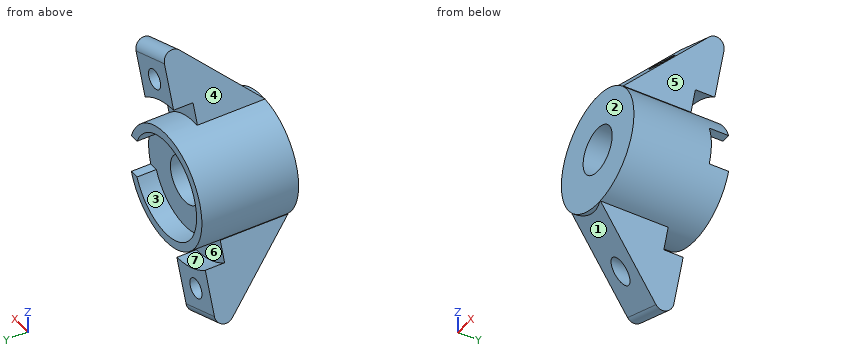
```python
from build123d import *

# Parameters (mm, degrees)
SKETCH1_R            = 12
SKETCH1_R_2          = 4.8
BOSS_EXTRUDE2_DEPTH  = 20
SKETCH1_3_R          = 4.8
CUT_EXTRUDE2_DEPTH   = 27.229754097
SKETCH3_R            = 10.25
CUT_EXTRUDE3_DEPTH   = 4
SKETCH5_W            = 11.035067707
SKETCH5_H            = 8
CUT_EXTRUDE5_DEPTH   = 4
BOSS_EXTRUDE3_DEPTH  = 5
SKETCH7_R            = 16.1
SKETCH7_R_2          = 12
CUT_EXTRUDE6_DEPTH   = 6
CUT_EXTRUDE7_REACH   = 39.1
SKETCH9_R            = 2
FILLET1_R            = 2
FILLET1_OF_MIRROR1_R = 2


with BuildPart() as part:
    # Sketch1 → Boss-Extrude2 (new body)
    # profile 1 of 2: a face of its own
    with BuildSketch(Plane(origin=(0, 0, 0), x_dir=(1, 0, 0), z_dir=(0, 1, 0))):
        with Locations(Location((0, 0, 0), (0, 0, 270))):
            Circle(SKETCH1_R)
        Circle(SKETCH1_R_2, mode=Mode.SUBTRACT)
    # profile 2 of 2: a face of its own
    with BuildSketch(Plane(origin=(0, 0, 0), x_dir=(1, 0, 0), z_dir=(0, 1, 0))):
        Circle(SKETCH1_R_2)
    extrude(amount=-BOSS_EXTRUDE2_DEPTH)

    # Sketch1<3> → Cut-Extrude2 (cut, through all)
    with BuildSketch(Plane(origin=(0, 0, 0), x_dir=(1, 0, 0), z_dir=(0, 1, 0))):
        with Locations(Location((0, 0, 0), (0, 0, 270))):
            Circle(SKETCH1_3_R)
    extrude(amount=-CUT_EXTRUDE2_DEPTH, mode=Mode.SUBTRACT)

    # Sketch3 → Cut-Extrude3 (cut)
    with BuildSketch(Plane(origin=(0, 0, 0), x_dir=(1, 0, 0), z_dir=(0, 1, 0))):
        with Locations(Location((0, 0, 0), (0, 0, 270))):
            Circle(SKETCH3_R)
    extrude(amount=-CUT_EXTRUDE3_DEPTH, mode=Mode.SUBTRACT)

    # Sketch5 → Cut-Extrude5 (cut)
    with BuildSketch(Plane(origin=(0, 0, 0), x_dir=(1, 0, 0), z_dir=(0, 1, 0))):
        with Locations((10.966087066, 0)):
            Rectangle(SKETCH5_W, SKETCH5_H)
    extrude(amount=-CUT_EXTRUDE5_DEPTH, mode=Mode.SUBTRACT)

    # Sketch6 → Boss-Extrude3 (add, symmetric)
    with BuildSketch(Plane(origin=(0, 0, 0), x_dir=(0, -1, 0), z_dir=(-0.9396926207859094, 0, 0.34202014332566616))):
        Polygon((2, -11), (20, -11), (2, -29), align=None)
    boss_extrude3 = extrude(amount=BOSS_EXTRUDE3_DEPTH, both=True)

    # Sketch7 → Cut-Extrude6 (cut)
    with BuildSketch(Plane(origin=(0, 0, 0), x_dir=(1, 0, 0), z_dir=(0, 1, 0))):
        Circle(SKETCH7_R)
        with Locations(Location((0, 0, 0), (0, 0, 340.528779366))):
            Circle(SKETCH7_R_2, mode=Mode.SUBTRACT)
    cut_extrude6 = extrude(amount=-CUT_EXTRUDE6_DEPTH, mode=Mode.SUBTRACT)

    # Cut-Extrude7: up to this plane
    cut_extrude7_end = Plane(origin=(0.936241527, -20, -12.046719545), z_dir=(-0.2418447626479747, -0.7071067811865439, -0.664463024388679))
    # Sketch9 → Cut-Extrude7 (cut, up to the surface)
    with BuildSketch(Plane(origin=(0, -2, 0), x_dir=(1, 0, 0), z_dir=(0, 1, 0)), mode=Mode.PRIVATE) as cut_extrude7_sk1:
        with Locations(Location((-6.840402867, 18.793852416, 0), (0, 0, 270))):
            Circle(SKETCH9_R)
    cut_extrude7_tool1 = split(extrude(cut_extrude7_sk1.sketch, amount=-CUT_EXTRUDE7_REACH, mode=Mode.PRIVATE), bisect_by=cut_extrude7_end, keep=Keep.BOTH, mode=Mode.PRIVATE)
    cut_extrude7 = cut_extrude7_tool1.solids().sort_by_distance((-6.840403, -2, -18.793852))[0]
    add(cut_extrude7, mode=Mode.SUBTRACT)

    # Fillet1
    fillet1_edges = [part.edges().sort_by_distance(p)[0] for p in [
        (-9.918584156, -2, -27.251086003),
    ]]
    fillet(fillet1_edges, radius=FILLET1_R)

    # Mirror1: Boss-Extrude3, Cut-Extrude6, Cut-Extrude7 across plane
    add(boss_extrude3.mirror(Plane(origin=(0, 0, 0), x_dir=(0.9396926207859094, 0, -0.3420201433256661), z_dir=(-0.3420201433256661, 0, -0.9396926207859093))))
    add(cut_extrude6.mirror(Plane(origin=(0, 0, 0), x_dir=(0.9396926207859094, 0, -0.3420201433256661), z_dir=(-0.3420201433256661, 0, -0.9396926207859093))), mode=Mode.SUBTRACT)
    add(cut_extrude7.mirror(Plane(origin=(0, 0, 0), x_dir=(0.9396926207859094, 0, -0.3420201433256661), z_dir=(-0.3420201433256661, 0, -0.9396926207859093))), mode=Mode.SUBTRACT)

    # Fillet1 of Mirror1
    fillet1_of_mirror1_edges = [part.edges().sort_by_distance(p)[0] for p in [
        (9.918584156, -2, 27.251086003),
    ]]
    fillet(fillet1_of_mirror1_edges, radius=FILLET1_OF_MIRROR1_R)


solid = part.part
```
The listing builds one solid part. Answer for the finished solid, in the listing's coordinates (mm). Face numbers are marked on the shaded views. A direction names the side the tool comes from. Coordinates: 2 decimals unless noted, no trailing zeros. Order: outer loops, then holes, each group sorted by start corner. A loop starts at its lowest first (then second) coordinate and runs counter-clockwise, first axis right, second up. Notation, with made-up numbers: M 72.25,-27.75 L 92.25,-27.75 A20 ccw 92.25,-6.75 Z; hole C -2,80 d2. An arc over 180 degrees is marked long. Answer as a JSON object with one key per item and string values. Group by question number.
1. Section D-D on z = -18 is taken. Write down the section's boundary in (x, y), then the cut area to 3 significant figures.
2. Determine the mould class of the marked faces 1, 2, 3 and 4 for opening direction Z: released by +Z, released by -Z, zero draft, split by the parting line, or undercut.
3. Straight lines are drawn through the part: line 1 (X direction, y = -13.75, z = 0); line 2 (Z direction, x = 4.5, y = -2.75); line 3 (Y direction, x = 5.75, z = -7.5). For each, find the intervals that lie inside material, in ascending order.
4. Flat-ended cylindrical pins translate along their axes: P1, Ø6.5, axis at x = 6.84, z = 18.79, coming from the -Y side; P2, Ø5, axis at y = -16, z = -17, coming from the +X side; P3, Ø1, axis at y = -12, z = 0, coming from the -X side; P4, Ø3.5, axis at x = -6.84, z = -18.79, coming from the +Y side. Find the tip coordinate at first contact, or state that the pin passes through.
5. Section B-B on x = 0 is taken. Write down the section's boundary in (y, z), then the cut area to 3 significant figures.
6. Section A-A on z = 0 is taken. Write down the section's boundary in (x, y), then the cut area to 3 significant figures.
7. A tool of negligible diameter and unlimited length cuts with its end or side. For the marked faces 5, 6 and 7, from which of +Z, -Z, +X, -X, +Y, -Y can it reach the whole face along a straight path? Write none if from no direction.
8. Section C-C on y = -10.5 is taken. Write down the section's boundary in (x, z).
Values follow:
{
 "1": {"outline": "M -11.87,-10.02 L -8.68,-11.12 L -8.68,-2 L -11.87,-2 Z; M -5,-12.37 L -1.23,-13.66 L -1.23,-2 L -5,-2 Z", "area": "69.0 mm2"},
 "2": {"face 1": "released by -Z", "face 2": "zero draft", "face 3": "undercut", "face 4": "released by +Z"},
 "3": {"line 1": "-12 to -4.8, 4.8 to 12", "line 2": "-11.12 to -9.21, 9.21 to 11.12, 15.46 to 25.75", "line 3": "-20 to -4"},
 "4": {"P1": "y = -14.25", "P2": "x = 0.04", "P3": "x = -12", "P4": "through"},
 "5": {"outline": "M -20,-12 L -19.72,-12 L -17.26,-14.62 L -6,-14.62 L -6,-12 L 0,-12 L 0,-10.25 L -4,-10.25 L -4,-4.8 L -20,-4.8 Z; M -20,4.8 L -4,4.8 L -4,10.25 L 0,10.25 L 0,12 L -6,12 L -6,14.62 L -17.26,14.62 L -19.72,12 L -20,12 Z", "area": "310 mm2"},
 "6": {"outline": "M -12,-20 L -4.8,-20 L -4.8,-4 L -10.25,-4 L -10.25,0 L -12,0 Z; M 4.8,-20 L 12,-20 L 12,-4 L 4.8,-4 Z", "area": "237 mm2"},
 "7": {"face 5": "+X, +Y, -Y", "face 6": "+Y", "face 7": "+X, +Y"},
 "8": {"outline": "M -11.71,-17.55 L -8.83,-18.6 A2 cw long -5.19,-19.93 L -2.31,-20.97 L 0.94,-12.05 L 0.74,-11.98 A12 ccw 8.27,8.7 L 8.46,8.63 L 11.71,17.55 L 8.83,18.6 A2 cw long 5.19,19.93 L 2.31,20.97 L -0.94,12.05 L -0.74,11.98 A12 ccw -8.27,-8.7 L -8.46,-8.63 Z; hole C 0,0 d9.6"}
}
